```python
from build123d import *

# Parameters (mm, degrees)
SKETCH1_R           = 1.15
BOSS_EXTRUDE1_DEPTH = 25
FILLET1_R           = 0.3
FILLET2_R           = 0.3
SKETCH2_R           = 1.25
BOSS_EXTRUDE2_DEPTH = 5
CHAMFER1_SIZE       = 0.3
FILLET3_R           = 0.3


with BuildPart() as part:
    # Sketch1 → Boss-Extrude1 (new body)
    with BuildSketch(Plane(origin=(0, 0, 0), x_dir=(1, 0, 0), z_dir=(0, 1, 0))):
        Polygon((-1.299038106, 2.25), (-2.598076211, 0), (-1.299038106, -2.25), (1.299038106, -2.25), (2.598076211, 0), (1.299038106, 2.25), align=None)
        with Locations(Location((0, 0, 0), (0, 0, 270))):
            Circle(SKETCH1_R, mode=Mode.SUBTRACT)
    extrude(amount=BOSS_EXTRUDE1_DEPTH)

    # Fillet1
    fillet1_edges = [part.edges().sort_by_distance(p)[0] for p in [
        (1.299038106, 12.5, -2.25),
        (2.598076211, 12.5, 0),
        (1.299038106, 12.5, 2.25),
        (-1.299038106, 12.5, 2.25),
        (-2.598076211, 12.5, 0),
        (-1.299038106, 12.5, -2.25),
    ]]
    fillet(fillet1_edges, radius=FILLET1_R)

    # Fillet2
    fillet2_edges = [part.edges().sort_by_distance(p)[0] for p in [
        (0, 0, -2.25),
        (0, 25, -2.25),
        (1.948557159, 0, -1.125),
        (1.948557159, 0, 1.125),
        (0, 0, 2.25),
        (-1.948557159, 0, 1.125),
        (-1.948557159, 0, -1.125),
        (1.275833025, 0, 2.209807621),
        (-1.275833025, 0, 2.209807621),
        (-2.55166605, 0, 0),
        (-1.275833025, 0, -2.209807621),
        (2.55166605, 0, 0),
        (1.275833025, 0, -2.209807621),
        (1.948557159, 25, -1.125),
        (-1.948557159, 25, -1.125),
        (-1.948557159, 25, 1.125),
        (0, 25, 2.25),
        (1.948557159, 25, 1.125),
        (1.275833025, 25, 2.209807621),
        (-1.275833025, 25, 2.209807621),
        (-2.55166605, 25, 0),
        (-1.275833025, 25, -2.209807621),
        (2.55166605, 25, 0),
        (1.275833025, 25, -2.209807621),
    ]]
    fillet(fillet2_edges, radius=FILLET2_R)

    # Sketch2 → Boss-Extrude2 (add)
    with BuildSketch(Plane.XZ):
        with Locations(Location((0, 0, 0), (0, 0, 90))):
            Circle(SKETCH2_R)
    extrude(amount=BOSS_EXTRUDE2_DEPTH)

    # Chamfer1
    chamfer1_edges = [part.edges().sort_by_distance(p)[0] for p in [
        (0, -5, -1.25),
        (0, 25, -1.15),
    ]]
    chamfer(chamfer1_edges, length=CHAMFER1_SIZE)

    # Fillet3
    fillet3_edges = [part.edges().sort_by_distance(p)[0] for p in [
        (0, 0, -1.25),
    ]]
    fillet(fillet3_edges, radius=FILLET3_R)


solid = part.part
```
For this review, take the finished solid that the model builds, in its own axes (mm). Give positions to 0.01 mm unless a question says otherwise; leave off trailing zeros. Write each loop counter-clockwise with the first axis right and the second up, starting at its lowest first coordinate (ties: lowest second). Pieces come first, ordered by that corner, then holes. Notation, with made-up numbers: M 32.25,83.5 L 77.25,83.5 A20 cw 77.25,107.5 Z; hole C 10,-19 d2. An arc over 180 degrees is marked long. One line per item, written item: value.
1) For P1, Ø2.5, axis at x = 0, z = 0.5, coming from the +Y side, flat-tipped, find the tip position at first contact; note if it passes through.
Results are:
P1: stops at y = 25
2) Take a section at B-B, the plane x = 0. Write out the cut boundary in (y, z).
Results are:
outline: M -5,-0.95 L -4.7,-1.25 L -0.3,-1.25 A0.3 cw 0,-1.55 L 0,-1.95 A0.3 ccw 0.3,-2.25 L 24.7,-2.25 A0.3 ccw 25,-1.95 L 25,-1.45 L 24.7,-1.15 L 0,-1.15 L 0,1.15 L 24.7,1.15 L 25,1.45 L 25,1.95 A0.3 ccw 24.7,2.25 L 0.3,2.25 A0.3 ccw 0,1.95 L 0,1.55 A0.3 cw -0.3,1.25 L -4.7,1.25 L -5,0.95 Z
3) The part is to be moulded in two halves that separate along Z. For faces 1 (the cylindrical face through (0.345, 12.177, 1.097)), 2 (the flat face through (0, 12, -2.25)), 3 (the cylindrical face through (1.22, -2.47, -0.27)), 4 (the flat face through (0, 0, 0)), say which applies: +Z half, -Z half, draft (parallel to the pull), parting line (faces both ways), or undercut.
Results are:
face 1: undercut
face 2: -Z half
face 3: parting line
face 4: undercut
4) Take a section at A-A, the plane y = 13.25. Write out the cut boundary in (x, z).
Results are:
outline: M -2.51,-0.15 L -1.39,-2.1 A0.3 ccw -1.13,-2.25 L 1.13,-2.25 A0.3 ccw 1.39,-2.1 L 2.51,-0.15 A0.3 ccw 2.51,0.15 L 1.39,2.1 A0.3 ccw 1.13,2.25 L -1.13,2.25 A0.3 ccw -1.39,2.1 L -2.51,0.15 A0.3 ccw Z; hole C 0,0 d2.3
5) For line 1 (X direction, y = 17, z = 0); line 2 (Y direction, x = -0.95, z = -1.5); line 3 (Z direction, x = -1, y = 6.25), list the stretches that pass through material, from the lowest coordinate up. Write a range as from..to.
Results are:
line 1: x = -2.55..-1.15, 1.15..2.55
line 2: y = 0..25
line 3: z = -2.25..-0.57, 0.57..2.25
6) Take a section at C-C, the plane y = -2.5. Write out the cut boundary in (x, z).
Results are:
outline: C 0,0 d2.5
